Input: part model. Units: mm. Frame: model coordinates. A direction names the side the tool comes from. Coordinates: 2 decimals unless noted, no trailing zeros. Loops run counter-clockwise (first coordinate to the right, second up) from the corner with the lowest first, then second, coordinate; pieces in that order, holes last. Notation, with made-up numbers: (8.5, -2.5) -> (48.5, -2.5) arc R23 cw to (48.5, 16.5) -> close; hole circle Ø5 at (17.25, 0.25). An arc over 180 degrees is marked (long way). Answer as a JSON object with one key per item and string values.
from build123d import *

# Parameters (mm, degrees)
SKETCH_1_R             = 120
EXTRUDE_1_DEPTH        = 50
EXTRUDE_1_2_DEPTH      = 50
EXTRUDE_1_2_DEPTH_BACK = 50
SKETCH_2_R             = 55
SKETCH_2_R_2           = 45
SKETCH_7_R             = 2
CUT_EXTRUDE_2_DEPTH    = 3
SKETCH_8_R             = 55
EXTRUDE_2_DEPTH        = 20
SKETCH_9_R             = 1.75
SKETCH_9_R_2           = 4
CUT_EXTRUDE_3_DEPTH    = 293.65045703


with BuildPart() as part:
    # 草图1 → Extrude 1 (new body)
    with BuildSketch(Plane(origin=(0, 0, 0), x_dir=(1, 0, 0), z_dir=(0, 1, 0))):
        with Locations(Location((0, 0, 0), (0, 0, 270))):
            Circle(SKETCH_1_R)
    extrude(amount=EXTRUDE_1_DEPTH)

    # 草图2 → Extrude 1 2 (add, two sides: drawn at the far end of the back side and taken through both)
    with BuildSketch(Plane.XY.offset(-EXTRUDE_1_2_DEPTH_BACK)):
        with Locations((0, 100)):
            Circle(SKETCH_2_R)
        with Locations((0, 100)):
            Circle(SKETCH_2_R_2, mode=Mode.SUBTRACT)
    extrude(amount=EXTRUDE_1_2_DEPTH + EXTRUDE_1_2_DEPTH_BACK)

    # 草图7 → 切除-拉伸2 (cut)
    with BuildSketch(Plane.XZ):
        with Locations(Location((17.25, 0, 0), (0, 0, 270))):
            Circle(SKETCH_7_R)
        with Locations(Location((8.625, -14.938938215, 0), (0, 0, 270))):
            Circle(SKETCH_7_R)
        with Locations(Location((-8.625, -14.938938215, 0), (0, 0, 270))):
            Circle(SKETCH_7_R)
        with Locations(Location((-17.25, 0, 0), (0, 0, 270))):
            Circle(SKETCH_7_R)
        with Locations(Location((-8.625, 14.938938215, 0), (0, 0, 270))):
            Circle(SKETCH_7_R)
        with Locations(Location((8.625, 14.938938215, 0), (0, 0, 270))):
            Circle(SKETCH_7_R)
    extrude(amount=-CUT_EXTRUDE_2_DEPTH, mode=Mode.SUBTRACT)

    # 草图8 → 凸台-拉伸2 (add)
    with BuildSketch(Plane.XY.offset(97.3)):
        with Locations((0, 100)):
            Circle(SKETCH_8_R)
    extrude(amount=EXTRUDE_2_DEPTH)

    # 草图9 → 切除-拉伸3 (cut, through all)
    with BuildSketch(Plane(origin=(0, 0, 97.3), x_dir=(-1, 0, 0), z_dir=(0, 0, -1))):
        with Locations((42.5, 100)):
            Circle(SKETCH_9_R)
        with Locations((30.0520382, 69.9479618)):
            Circle(SKETCH_9_R)
        with Locations((0, 57.5)):
            Circle(SKETCH_9_R)
        with Locations((-30.0520382, 69.9479618)):
            Circle(SKETCH_9_R)
        with Locations((-42.5, 100)):
            Circle(SKETCH_9_R)
        with Locations((-30.0520382, 130.0520382)):
            Circle(SKETCH_9_R)
        with Locations((0, 142.5)):
            Circle(SKETCH_9_R)
        with Locations((30.0520382, 130.0520382)):
            Circle(SKETCH_9_R)
        with Locations((0, 100)):
            Circle(SKETCH_9_R_2)
    extrude(amount=-CUT_EXTRUDE_3_DEPTH, mode=Mode.SUBTRACT)


solid = part.part
1. Access query for faces 1 (the face through (5.276, 24.65, -119.884)), 2 (the face through (-9.76, 56.07, -0.7)), 3 (the face through (-25, 138, 50)), 4 (the face through (-1.846, 96.451, 107.16)). Directions: +Z, -Z, +X, -X, +Y, -Y. A direction counts if a zero-diameter tool reaches every point of the face in a straight line with its end or side. Return the directions, or none.
Reply:
{"face 1": "-Y", "face 2": "-Z", "face 3": "+X, -X, +Y", "face 4": "+Z, -Z"}
2. Pin query (flat end, axial travel): P1, Ø10, axis at x = 23.5, z = -12, coming from the +Y side; P2, Ø3, axis at x = -17.25, z = 0, coming from the -Y side; P3, Ø4.5, axis at x = -30.05, y = 130.05, coming from the +Z side. Return the tip coordinate at first contact, or that it passes through.
Reply:
{"P1": "stops at y = 151.8", "P2": "stops at y = 3", "P3": "stops at z = 117.3"}
3. Line query: line 1 along X through (y, z) = (1.2, 0); line 2 along Y through (x, z) = (0, 111); line 3 along Z through (x, y) = (48, 93). Output: solid intervals per line, ascending.
Reply:
{"line 1": "x = -120 to -19.25, -15.25 to 15.25, 19.25 to 120", "line 2": "y = 0 to 55.75, 59.25 to 96, 104 to 140.75, 144.25 to 155", "line 3": "z = -50 to 50, 97.3 to 117.3"}
4. Mould query, pull axis Z, two halves, no side actions, for faces 5 (the face through (2, 0, -2)), 6 (the face through (-1, 92, 97.3)), 7 (the face through (-25, 138, -50)), 8 (the face through (-1, 92, 117.3)). Classes: pulls with the +Z half, pulls with the -Z half, needs draft (parallel to the pull), parting line crosses it, or undercut.
Reply:
{"face 5": "needs draft", "face 6": "undercut", "face 7": "pulls with the -Z half", "face 8": "pulls with the +Z half"}
5. Section query C-C (y = 10.5). Return loops of the section in (x, z).
Reply:
{"outline": "circle Ø240 at (0, 0)"}
6. Section query D-D (x = 74). Return loops of the section in (y, z), plus the area to 3 significant figures.
Reply:
{"outline": "(0, -94.47) -> (50, -94.47) -> (50, 94.47) -> (0, 94.47) -> close", "area": "9,450 mm2"}
7. Section query A-A (z = 103). Count the separate pieces of the cut face and the enclosed holes in it, plus the area to 3 significant figures.
Reply:
{"separate pieces": "1", "enclosed holes": "9", "area": "15,400 mm2"}
8. Section query B-B (z = -25). Return loops of the section in (x, y), plus the area to 3 significant figures.
Reply:
{"outline": "(-117.37, 0) -> (117.37, 0) -> (117.37, 50) -> (22.91, 50) arc R55 ccw (long way) to (-22.91, 50) -> (-117.37, 50) -> close; hole circle Ø90 at (0, 100)", "area": "14,700 mm2"}
